Check sheet for the modelled part. Datum: model origin and axes. Units: mm. Give positions to 0.01 mm unless a question says otherwise; leave off trailing zeros. Order: outer loops, then holes, each group sorted by start corner. A loop starts at its lowest first (then second) coordinate and runs counter-clockwise, first axis right, second up. Notation, with made-up numbers: (-40, -21) -> (17, -21) arc R24 cw to (17, 13) -> close; hole circle Ø5 at (89.25, -16). An arc over 180 degrees is marked (long way). Answer in a Markdown table with one row per item. Add a question column.
(1) Cross-section at A-A (y = 22.5). Record the cut outline in (x, z) (3 decimals), then the cut area to 3 significant figures.
(2) Cross-section at C-C (z = -12.5). Record the cut outline in (x, y).
(3) Cross-section at B-B (z = 3). Record the cut outline in (x, y).
(4) Thickness scan on L1, parallel to Z at x = -37, y = 16.5; L2, parallel to X at y = 19, z = -9.5. Record the ranges inside material, lowest first. Write a range as [from, to].
(5) Go/stop test with flat-tipped pins: pin 1 (1.9 mm diameter, centred on x = -41, z = 0.5, fed in from -Y); pin 2 (6 mm diameter, centred on y = 4.5, z = -1.5, fed in from -X); pin 3 (1.4 mm diameter, centred on x = -41.5, y = 36, fed in from -Z). Record where each tip stops, or that it passes through.
```python
from build123d import *

# Parameters (mm, degrees)
SKETCH1_W           = 76.2
SKETCH1_H           = 39.37
BOSS_EXTRUDE1_DEPTH = 38.1
SKETCH2_W           = 12.7
SKETCH2_H           = 3.81
BOSS_EXTRUDE2_DEPTH = 5.08
FILLET1_R           = 1.27


with BuildPart() as part:
    # Sketch1 → Boss-Extrude1 (new body)
    with BuildSketch(Plane(origin=(0, 0, 0), x_dir=(1, 0, 0), z_dir=(0, 1, 0))):
        Rectangle(SKETCH1_W, SKETCH1_H)
    extrude(amount=BOSS_EXTRUDE1_DEPTH)

    # Sketch2 → Boss-Extrude2 (add)
    with BuildSketch(Plane.ZY.offset(38.1)):
        with Locations((0, 36.195)):
            Rectangle(SKETCH2_W, SKETCH2_H)
    extrude(amount=BOSS_EXTRUDE2_DEPTH)

    # Fillet1
    fillet1_edges = [part.edges().sort_by_distance(p)[0] for p in [
        (-38.1, 38.1, -13.0175),
        (-38.1, 38.1, 13.0175),
        (-38.1, 36.195, -6.35),
        (-40.64, 38.1, -6.35),
        (-38.1, 34.29, 0),
        (0, 38.1, 19.685),
        (-40.64, 34.29, -6.35),
        (-38.1, 36.195, 6.35),
        (-40.64, 34.29, 6.35),
        (-40.64, 38.1, 6.35),
        (38.1, 38.1, 0),
        (0, 0, 19.685),
        (-38.1, 0, 0),
        (0, 0, -19.685),
        (38.1, 0, 0),
        (38.1, 19.05, 19.685),
        (-38.1, 19.05, 19.685),
        (-38.1, 19.05, -19.685),
        (38.1, 19.05, -19.685),
        (0, 38.1, -19.685),
    ]]
    fillet(fillet1_edges, radius=FILLET1_R)


solid = part.part
```
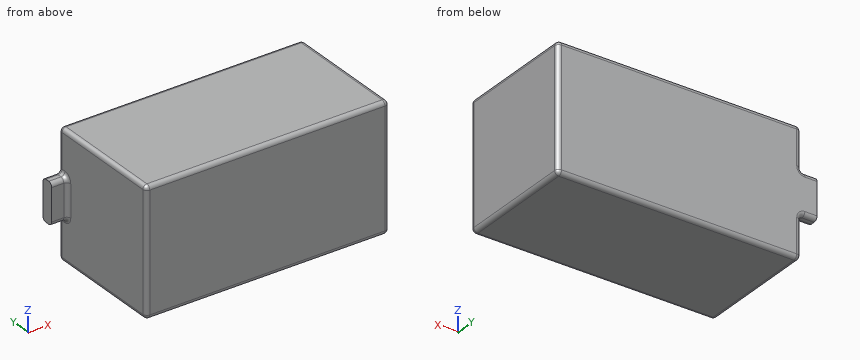
Answer below:
| question | item | result |
|---|---|---|
| 1 | outline | (-38.1, -18.415) arc R1.27 ccw to (-36.83, -19.685) -> (36.83, -19.685) arc R1.27 ccw to (38.1, -18.415) -> (38.1, 18.415) arc R1.27 ccw to (36.83, 19.685) -> (-36.83, 19.685) arc R1.27 ccw to (-38.1, 18.415) -> close |
| 1 | area | 3,000 mm² |
| 2 | outline | (-38.1, 1.27) arc R1.27 ccw to (-36.83, 0) -> (36.83, 0) arc R1.27 ccw to (38.1, 1.27) -> (38.1, 36.83) arc R1.27 ccw to (36.83, 38.1) -> (-36.83, 38.1) arc R1.27 ccw to (-38.1, 36.83) -> close |
| 3 | outline | (-43.18, 34.29) -> (-39.37, 34.29) arc R1.27 cw to (-38.1, 33.02) -> (-38.1, 1.27) arc R1.27 ccw to (-36.83, 0) -> (36.83, 0) arc R1.27 ccw to (38.1, 1.27) -> (38.1, 36.83) arc R1.27 ccw to (36.83, 38.1) -> (-43.18, 38.1) -> close |
| 4 | L1 | z = [-19.67, 19.67] |
| 4 | L2 | x = [-38.1, 38.1] |
| 5 | pin 1 | stops at y = 34.29 |
| 5 | pin 2 | stops at x = -38.1 |
| 5 | pin 3 | stops at z = -6.35 |
